Part model, mm, in its own coordinate system. Face numbers are marked on the shaded views. A direction names the side the tool comes from. Coordinates: 2 decimals unless noted, no trailing zeros. Write each loop counter-clockwise with the first axis right and the second up, starting at its lowest first coordinate (ties: lowest second). Pieces come first, ordered by that corner, then holes. Notation, with made-up numbers: (28.25, 23.25) -> (42.25, 23.25) arc R25 ccw to (42.25, 52.25) -> close; hole circle Ø5 at (9, 77.25). An arc over 180 degrees is marked (long way). Write item = value, one per line. Start each with the question number.
Q1. Tool access for the marked faces 4, 5 and 6: list every direction of +Z, -Z, +X, -X, +Y, -Y with a clear straight run to the whole face (end or side of a thin tool).
Q2. Probe line 1 (X direction, y = 0.95, z = -7); line 2 (Z direction, x = 2.5, y = 1.25); line 3 (X direction, y = 0.15, z = -6.25). List the from-to ranges inside material, lowest first.
Q3. Band-saw the part on A-A, the plane z = -7. List the corners of the cut face in (x, y).
Q4. Band-saw the part on B-B, the plane x = 8.25. List the corners of the cut face in (y, z).
Q5. Pin check, flat tips, straight feed: P1, Ø0.6, axis at y = 1, z = -10.5, coming from the +X side; P2, Ø2.5, axis at x = 2.5, z = -7, coming from the +Y side. Stop position of each tip, or through.
Q6. Pull direction X, two halves, no side cores. Call the marked faces 1, 2 and 3: released by +X, released by -X, zero draft, split by the parting line, or undercut.
Q7. Band-saw the part on C-C, the plane y = 1.2. List the corners of the cut face in (x, z), plus the area to 3 significant figures.
Q8. Band-saw the part on D-D, the plane z = -2.5. List the corners of the cut face in (x, y), plus the area to 3 significant figures.
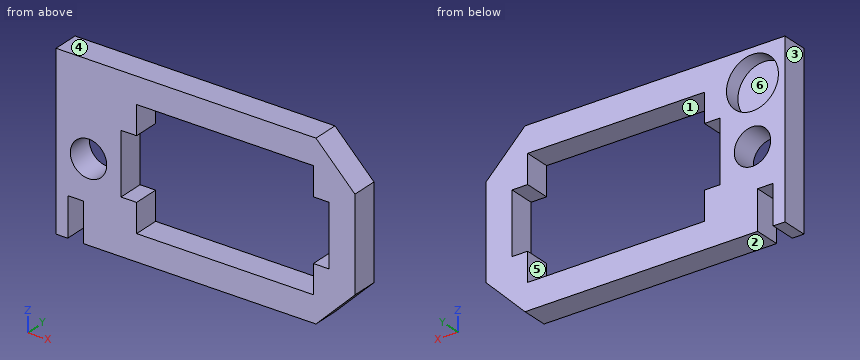
from build123d import *

# Parameters (mm, degrees)
ESQUISSE1_W             = 23
ESQUISSE1_H             = 13.1
BOSS_EXTRU_1_DEPTH      = 2
ENL_V_MAT_EXTRU_4_REACH = 4
ESQUISSE2_R             = 1.4
CHANFREIN1_SIZE         = 3
ESQUISSE3_W             = 1.2
ESQUISSE3_H             = 2
ENL_V_MAT_EXTRU_5_DEPTH = 3
ESQUISSE4_R             = 2
ENL_V_MAT_EXTRU_6_DEPTH = 1.2


with BuildPart() as part:
    # Esquisse1 → Boss.-Extru.1 (new body)
    with BuildSketch(Plane(origin=(0, 0, 0), x_dir=(1, 0, 0), z_dir=(0, 1, 0))):
        with Locations((11.5, 6.55)):
            Rectangle(ESQUISSE1_W, ESQUISSE1_H)
        Polygon((6.2, 8.9), (6.2, 11.1), (19.8, 11.1), (19.8, 8.9), (21, 8.9), (21, 4.2), (19.8, 4.2), (19.8, 2), (6.2, 2), (6.2, 4.2), (5, 4.2), (5, 8.9), align=None, mode=Mode.SUBTRACT)
    extrude(amount=BOSS_EXTRU_1_DEPTH)

    # Esquisse2 → Enlèv. mat.-Extru.4 (cut, up to next)
    with BuildSketch(Plane(origin=(0, 2, 0), x_dir=(1, 0, 0), z_dir=(0, 1, 0)), mode=Mode.PRIVATE) as enl_v_mat_extru_4_sk1:
        with Locations((2.5, 7)):
            Circle(ESQUISSE2_R)
    enl_v_mat_extru_4_tool1 = extrude(enl_v_mat_extru_4_sk1.sketch, amount=-ENL_V_MAT_EXTRU_4_REACH, mode=Mode.PRIVATE) & part.part
    add(enl_v_mat_extru_4_tool1.solids().sort_by_distance((2.5, 2, -7))[0], mode=Mode.SUBTRACT)

    # Chanfrein1
    chanfrein1_edges = [part.edges().sort_by_distance(p)[0] for p in [
        (23, 1, -13.1),
        (23, 1, 0),
    ]]
    chamfer(chanfrein1_edges, length=CHANFREIN1_SIZE)

    # Esquisse3 → Enlèv. mat.-Extru.5 (cut)
    with BuildSketch(Plane(origin=(0, 0, -13.1), x_dir=(-1, 0, 0), z_dir=(0, 0, -1))):
        with Locations((-1.5, 1)):
            Rectangle(ESQUISSE3_W, ESQUISSE3_H)
    extrude(amount=-ENL_V_MAT_EXTRU_5_DEPTH, mode=Mode.SUBTRACT)

    # Esquisse4 → Enlèv. mat.-Extru.6 (cut)
    with BuildSketch(Plane(origin=(0, 2, 0), x_dir=(1, 0, 0), z_dir=(0, 1, 0))):
        with Locations((2.5, 2.5)):
            Circle(ESQUISSE4_R)
    extrude(amount=-ENL_V_MAT_EXTRU_6_DEPTH, mode=Mode.SUBTRACT)


solid = part.part
Ans:
q1.face_4 = +Z, +X, -X, +Y, -Y
q1.face_5 = +Y, -Y
q1.face_6 = +Y
q2.line_1 = 0 to 1.1, 3.9 to 5, 21 to 23
q2.line_2 = -13.1 to -8.4, -5.6 to -4.5, -0.5 to 0
q2.line_3 = 0 to 1.32, 3.68 to 5, 21 to 23
q3.outline = (0, 0) -> (1.1, 0) -> (1.1, 2) -> (0, 2) -> close; (3.9, 0) -> (5, 0) -> (5, 2) -> (3.9, 2) -> close; (21, 0) -> (23, 0) -> (23, 2) -> (21, 2) -> close
q4.outline = (0, -13.1) -> (2, -13.1) -> (2, -11.1) -> (0, -11.1) -> close; (0, -2) -> (2, -2) -> (2, 0) -> (0, 0) -> close
q5.P1 = 22.9
q5.P2 = through
q6.face_1 = undercut
q6.face_2 = zero draft
q6.face_3 = released by -X
q7.outline = (0, -13.1) -> (0.9, -13.1) -> (0.9, -10.1) -> (2.1, -10.1) -> (2.1, -13.1) -> (20, -13.1) -> (23, -10.1) -> (23, -3) -> (20, 0) -> (0, 0) -> close; hole circle Ø4 at (2.5, -2.5); hole circle Ø2.8 at (2.5, -7); hole (5, -8.9) -> (6.2, -8.9) -> (6.2, -11.1) -> (19.8, -11.1) -> (19.8, -8.9) -> (21, -8.9) -> (21, -4.2) -> (19.8, -4.2) -> (19.8, -2) -> (6.2, -2) -> (6.2, -4.2) -> (5, -4.2) -> close
q7.area = 135 mm2
q8.outline = (0, 0) -> (6.2, 0) -> (6.2, 2) -> (4.5, 2) -> (4.5, 0.8) -> (0.5, 0.8) -> (0.5, 2) -> (0, 2) -> close; (19.8, 0) -> (22.5, 0) -> (22.5, 2) -> (19.8, 2) -> close
q8.area = 13.0 mm2
